Build history of the part. All positions in model axes, mm. A direction names the side the tool comes from. Give positions to 0.01 mm unless a question says otherwise; leave off trailing zeros. Order: outer loops, then holes, each group sorted by start corner. A loop starts at its lowest first (then second) coordinate and runs counter-clockwise, first axis right, second up. Notation, with made-up numbers: M -16.75,79.25 L -9.75,79.25 A19 cw -9.75,85.25 Z; hole C 28,-39.5 d11. An arc over 180 degrees is marked long. One line per item, written item: value. Start each with the question number.
from build123d import *

# Parameters (mm, degrees)
F0_W     = 38.1
F0_H     = 38.1
F0_R     = 3.81
F0_R_2   = 12.7635
F1_DEPTH = 114.3
F2_R     = 12.7635
F2_R_2   = 1.75
F3_DEPTH = 10.1


with BuildPart() as f1:
    # F0 (on Front) → F1 (new body)
    with BuildSketch(Plane.XZ):
        Rectangle(F0_W, F0_H)
        with Locations((-12.7, -12.7)):
            Circle(F0_R, mode=Mode.SUBTRACT)
        with Locations((12.7, -12.7)):
            Circle(F0_R, mode=Mode.SUBTRACT)
        with Locations((-12.7, 12.7)):
            Circle(F0_R, mode=Mode.SUBTRACT)
        Circle(F0_R_2, mode=Mode.SUBTRACT)
        with Locations((12.7, 12.7)):
            Circle(F0_R, mode=Mode.SUBTRACT)
    extrude(amount=F1_DEPTH)

    # F2 (on face) → F3 (join)
    with BuildSketch(Plane.XZ.offset(114.3)):
        Circle(F2_R)
        Circle(F2_R_2, mode=Mode.SUBTRACT)
    extrude(amount=-F3_DEPTH)


solid = f1.part
1) Pull direction Z, two halves, no side cores. Call faces 3 (the cylindrical face through (-13.53, -56.35, -16.42)), 4 (the flat face through (0, 0, 13)), 5 (the flat face through (0, -56, 19.05)), 6 (the cylindrical face through (-16.506, -56.35, 12.868)): pulls with the +Z half, pulls with the -Z half, needs draft (parallel to the pull), parting line crosses it, or undercut.
2) Slice it at B-B (x = 0). List the corners of the cut face in (y, z).
3) Tool access for faces 1 (the flat face through (3, -104.2, 0)), 2 (the flat face through (19.05, -56, 0)): list every direction of +Z, -Z, +X, -X, +Y, -Y with a clear straight run to the whole face (end or side of a thin tool).
4) Slice it at C-C (y = -80). List the corners of the cut face in (x, z).
5) Drill centre lines: line 1 (Z direction, x = -11.5, y = -35); line 2 (Z direction, x = 0, y = -70.5); line 3 (X direction, y = -61, z = 14). Where is each one in solid material? Low to high.
6) Slice it at D-D (z = 10.5). List the corners of the cut face in (x, y).
7) Slice it at A-A (z = 0). List the corners of the cut face in (x, y).
8) Drop a flat-ended pin along its axis: P1, Ø20.5, axis at x = 0, z = 0, coming from the +Y side. Give the stop position or say it passes through.
Results list:
1. face 3: undercut
1. face 4: needs draft
1. face 5: pulls with the +Z half
1. face 6: undercut
2. outline: M -114.3,-19.05 L 0,-19.05 L 0,-12.76 L -104.2,-12.76 L -104.2,-1.75 L -114.3,-1.75 Z; M -114.3,1.75 L -104.2,1.75 L -104.2,12.76 L 0,12.76 L 0,19.05 L -114.3,19.05 Z
3. face 1: +Y
3. face 2: +Z, -Z, +X, +Y, -Y
4. outline: M -19.05,-19.05 L 19.05,-19.05 L 19.05,19.05 L -19.05,19.05 Z; hole C -12.7,-12.7 d7.62; hole C -12.7,12.7 d7.62; hole C 0,0 d25.53; hole C 12.7,-12.7 d7.62; hole C 12.7,12.7 d7.62
5. line 1: z = -19.05 to -16.32, -9.08 to -5.54, 5.54 to 9.08, 16.32 to 19.05
5. line 2: z = -19.05 to -12.76, 12.76 to 19.05
5. line 3: x = -19.05 to -16.28, -9.12 to 9.12, 16.28 to 19.05
6. outline: M -19.05,-114.3 L -15.81,-114.3 L -15.81,0 L -19.05,0 Z; M -9.59,-114.3 L 9.59,-114.3 L 9.59,0 L 7.26,0 L 7.26,-104.2 L -7.26,-104.2 L -7.26,0 L -9.59,0 Z; M 15.81,-114.3 L 19.05,-114.3 L 19.05,0 L 15.81,0 Z
7. outline: M -19.05,-114.3 L -1.75,-114.3 L -1.75,-104.2 L -12.76,-104.2 L -12.76,0 L -19.05,0 Z; M 1.75,-114.3 L 19.05,-114.3 L 19.05,0 L 12.76,0 L 12.76,-104.2 L 1.75,-104.2 Z
8. P1: stops at y = -104.2
